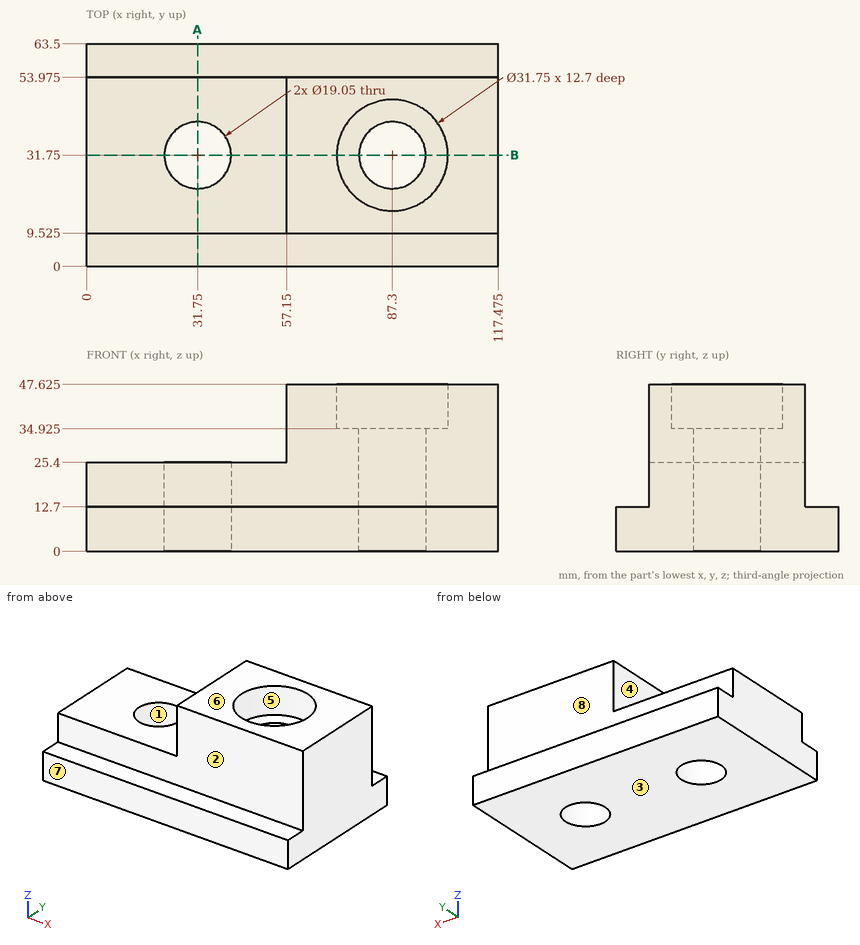
Here's the drawing with two shaded views (mm, measured from the low corner). I have some questions. A direction names the side the tool comes from. Give positions to 0.01 mm unless a question says otherwise; leave off trailing zeros. Order: outer loops, then holes, each group sorted by start corner. A loop starts at its lowest first (then second) coordinate and runs counter-clockwise, first axis right, second up. Notation, with made-up numbers: (31.5, -16) -> (71.5, -16) arc R19 cw to (71.5, 17) -> close; hole circle Ø2 at (85.25, 59). An arc over 180 degrees is marked (long way). One line per item, written item: value. Start each with the question number.
1. Will these pins go through, and if not, where does the flat tip stop? pin 1 Ø7.5 at (x, y) = (43, 4) entering from +Z; pin 2 Ø18 at (y, z) = (27, 36) entering from -X; pin 3 Ø9.5 at (x, y) = (79.5, 24.5) entering from +Z (3 decimals).
2. We'd pull the mould along Y, two halves only. Please class the marked faces 1, 2 and 3: released by +Y, released by -Y, zero draft, split by the parting line, or undercut.
3. For the marked faces 4, 5, 6, 7 and 8, which set-ups out of +Z, -Z, +X, -X, +Y, -Y let a thin tool reach every point of the face, with its end or its side?
4. I need wall thicknesses on probe 1 along X at (y, z) = (31.5, 25) (1 decimal); probe 2 along X at (y, z) = (23.5, 25) (1 decimal); probe 3 along Z at (x, y) = (7, 25.5). Which ranges of each line are inside material? Lowest first, please. Write a range as from..to.
5. Imagine slicing it at B-B, the plane y = 31.75. Count the separate pieces of the cut face and the enclosed holes in it, plus the area to 3 significant figures.
6. Imagine slicing it at A-A, the plane x = 31.75. List the corners of the cut face in (y, z) for me (3 decimals).
Values follow:
1. pin 1: stops at z = 12.7
1. pin 2: stops at x = 57.15
1. pin 3: stops at z = 34.925
2. face 1: undercut
2. face 2: released by -Y
2. face 3: zero draft
3. face 4: +Z, -X, +Y, -Y
3. face 5: +Z
3. face 6: +Z, +X, -X, +Y, -Y
3. face 7: +Z, -Z, +X, -X, -Y
3. face 8: +Z, +X, -X, +Y
4. probe 1: x = 0..22.2, 41.3..77.8, 96.8..117.5
4. probe 2: x = 0..27, 36.5..82.5, 92.1..117.5
4. probe 3: z = 0..25.4
5. separate pieces: 3
5. enclosed holes: 0
5. area: 2,770 mm2
6. outline: (0, 0) -> (22.225, 0) -> (22.225, 25.4) -> (9.525, 25.4) -> (9.525, 12.7) -> (0, 12.7) -> close; (41.275, 0) -> (63.5, 0) -> (63.5, 12.7) -> (53.975, 12.7) -> (53.975, 25.4) -> (41.275, 25.4) -> close
